from build123d import *

# Parameters (mm, degrees)
F0_W      = 50.8
F0_H      = 50.8
F1_DEPTH  = 7.62
F2_T      = -1.27
F3_W      = 1.27
F3_H      = 21.299569
F3_H_2    = 24.274384
F3_H_3    = 19.340431
F4_DEPTH  = 7.62
F5_W      = 10.16
F5_H      = 1.27
F5_W_2    = 15.24
F5_H_2    = 2.170816
F5_W_3    = 7.62
F5_R      = 3.81
F5_W_4    = 1.27
F5_H_3    = 19.382268
F6_DEPTH  = 7.62
F7_R      = 0.635
F8_DEPTH  = 25.4
F9_R      = 1.27
F10_DEPTH = 25.4
F11_R     = 1.27
F12_DEPTH = 25.4
F13_R     = 1.27
F14_DEPTH = 25.4
F15_DEPTH = 25.4
F16_W     = 1.27
F16_H     = 3.036126
F17_DEPTH = 7.62


with BuildPart() as f1:
    # F0 (on Top) → F1 (new body)
    with BuildSketch(Plane.XY):
        with Locations((25.4, 25.4)):
            Rectangle(F0_W, F0_H)
    extrude(amount=F1_DEPTH)

    # F2
    f2_openings = [f1.faces().sort_by_distance(p)[0] for p in [
        (25.4, 25.4, 7.62),
    ]]
    offset(amount=F2_T, openings=f2_openings)

    # F3 (on Top) → F4 (join)
    with BuildSketch(Plane.XY):
        with Locations((6.985, 10.649784)):
            Rectangle(F3_W, F3_H)
        with Locations((6.985, 38.516761)):
            Rectangle(F3_W, F3_H_2)
        with Locations((12.065, 36.049785)):
            Rectangle(F3_W, F3_H_3)
    extrude(amount=F4_DEPTH)

    # F5 (on Top) → F6 (join)
    with BuildSketch(Plane.XY):
        with Locations((44.073429, 7.922732)):
            Rectangle(F5_W, F5_H)
        with Locations((25.4, 40.315118)):
            Rectangle(F5_W_2, F5_H_2)
        with Locations((16.51, 14.74529)):
            Rectangle(F5_W_3, F5_H)
        with Locations((32.407153, 29.305989)):
            Circle(F5_R)
        with Locations((26.219592, 9.691134)):
            Rectangle(F5_W_4, F5_H_3)
    extrude(amount=F6_DEPTH)

    # F7 (on Top) → F8 (cut)
    with BuildSketch(Plane.XY):
        with Locations((3.863793, 5.102679)):
            Circle(F7_R)
    extrude(amount=-F8_DEPTH, mode=Mode.SUBTRACT)

    # F9 (on face) → F10 (cut)
    with BuildSketch(Plane.XY.offset(1.27)):
        with Locations((43.868799, 15.38029)):
            Circle(F9_R)
    extrude(amount=-F10_DEPTH, mode=Mode.SUBTRACT)

    # F11 (on face) → F12 (cut)
    with BuildSketch(Plane.XY.offset(1.27)):
        with Locations((38.372144, 37.351608)):
            Circle(F11_R)
    extrude(amount=-F12_DEPTH, mode=Mode.SUBTRACT)

    # F13 (on face) → F14 (cut)
    with BuildSketch(Plane.XY.offset(1.27)):
        with Locations((19.05, 32.861251)):
            Circle(F13_R)
        with Locations((4.185437, 47.093425)):
            Circle(F13_R)
        with Locations((4.185437, 6.017732)):
            Circle(F13_R)
    extrude(amount=-F14_DEPTH, mode=Mode.SUBTRACT)

    # F13 (on face) → F15 (cut)
    with BuildSketch(Plane.XY.offset(1.27)):
        with Locations((19.05, 32.861251)):
            Circle(F13_R)
        with Locations((4.185437, 47.093425)):
            Circle(F13_R)
        with Locations((4.185437, 6.017732)):
            Circle(F13_R)
    extrude(amount=-F15_DEPTH, mode=Mode.SUBTRACT)

    # F16 (on Top) → F17 (join)
    with BuildSketch(Plane.XY):
        with Locations((17.742798, 7.868063)):
            Rectangle(F16_W, F16_H)
    extrude(amount=F17_DEPTH)


solid = f1.part
Verification items for the finished model (mm, model axes). A direction names the side the tool comes from. Coordinates: 2 decimals unless noted, no trailing zeros. Order: outer loops, then holes, each group sorted by start corner. A loop starts at its lowest first (then second) coordinate and runs counter-clockwise, first axis right, second up.
Item 1: Access from +Z, -Z, +X, -X, +Y, -Y to the whole of each face (thin tool, end or side, straight path). Record for faces 4 (the face through (32, 29, 7.62)), 5 (the face through (20.32, 15, 4)).
Filled in:
face 4: +Z, +X, -X, +Y, -Y
face 5: +Z
Item 2: Section check D-D, the plane z = 3. Give the number of separate pieces and of enclosed holes in the cut face, then the cut area to 3 significant figures.
Filled in:
separate pieces: 7
enclosed holes: 1
area: 459 mm2
Item 3: Material ranges on L1, parallel to X at y = 43.5, z = 5.5; L2, parallel to X at y = 15, z = 4.25; L3, parallel to Y at x = 11.5, z = 2.25, recorded low to high.
Filled in:
L1: x = 0 to 1.27, 6.35 to 7.62, 11.43 to 12.7, 49.53 to 50.8
L2: x = 0 to 1.27, 6.35 to 7.62, 12.7 to 20.32, 25.58 to 26.85, 49.53 to 50.8
L3: y = 0 to 1.27, 26.38 to 45.72, 49.53 to 50.8
Item 4: Release check for a two-part mould opening along X. For faces 1 (the face through (49.53, 25, 4)), 2 (the face through (4, 1.27, 4)), 3 (the face through (25, 40, 7.62)) record: +X half, -X half, draft (parallel to the pull), parting line (faces both ways), or undercut.
Filled in:
face 1: undercut
face 2: undercut
face 3: draft
Item 5: Section check C-C, the plane x = 31.5. Enter the section's corners in (y, z), then the cut area to 3 significant figures.
Filled in:
outline: (0, 0) - (50.8, 0) - (50.8, 7.62) - (49.53, 7.62) - (49.53, 1.27) - (41.4, 1.27) - (41.4, 7.62) - (39.23, 7.62) - (39.23, 1.27) - (33.01, 1.27) - (33.01, 7.62) - (25.61, 7.62) - (25.61, 1.27) - (1.27, 1.27) - (1.27, 7.62) - (0, 7.62) - close
area: 141 mm2
Item 6: Depth check by flat-ended pin: pin 1 (1 mm diameter, centred on y = 8, z = 5.5, fed in from -X). Enter the tip coordinate at first touch or a pass-through.
Filled in:
pin 1: stops at x = 0
Item 7: Section check A-A, the plane x = 19.05. Enter the section's corners in (y, z).
Filled in:
outline: (0, 0) - (31.59, 0) - (31.59, 1.27) - (15.38, 1.27) - (15.38, 7.62) - (14.11, 7.62) - (14.11, 1.27) - (1.27, 1.27) - (1.27, 7.62) - (0, 7.62) - close; (34.13, 0) - (50.8, 0) - (50.8, 7.62) - (49.53, 7.62) - (49.53, 1.27) - (41.4, 1.27) - (41.4, 7.62) - (39.23, 7.62) - (39.23, 1.27) - (34.13, 1.27) - close
Item 8: Section check B-B, the plane y = 12.5. Enter the section's corners in (x, z).
Filled in:
outline: (0, 0) - (50.8, 0) - (50.8, 7.62) - (49.53, 7.62) - (49.53, 1.27) - (26.85, 1.27) - (26.85, 7.62) - (25.58, 7.62) - (25.58, 1.27) - (7.62, 1.27) - (7.62, 7.62) - (6.35, 7.62) - (6.35, 1.27) - (1.27, 1.27) - (1.27, 7.62) - (0, 7.62) - close
